```python
from build123d import *

# Parameters (mm, degrees)
EXTRUDE_1_DEPTH = 2697
SKETCH_2_W      = 61
SKETCH_2_H      = 134
EXTRUDE_2_DEPTH = 6
SKETCH_3_W      = 61
SKETCH_3_H      = 134
EXTRUDE_3_DEPTH = 6


with BuildPart() as part:
    # Model → 凸台-拉伸1 (new body)
    with BuildSketch(Plane.XY):
        with BuildLine():
            Line((11739.240027423, -58278.413223948), (11736.240027423, -58275.413223948))
            Line((11736.240027423, -58275.413223948), (11691.240027423, -58275.413223948))
            Line((11691.240027423, -58275.413223948), (11688.240027423, -58278.413223948))
            Line((11688.240027423, -58278.413223948), (11681.240027423, -58278.413223948))
            Line((11681.240027423, -58278.413223948), (11681.240027423, -58270.413223948))
            Line((11681.240027423, -58270.413223948), (11739.240027423, -58270.413223948))
            ThreePointArc((11739.240027423, -58270.413223948), (11741.361347766, -58269.534544291), (11742.240027423, -58267.413223948))
            Line((11742.240027423, -58267.413223948), (11742.240027423, -58139.413223948))
            ThreePointArc((11742.240027423, -58139.413223948), (11741.361347766, -58137.291903604), (11739.240027423, -58136.413223948))
            Line((11739.240027423, -58136.413223948), (11681.240027423, -58136.413223948))
            Line((11681.240027423, -58136.413223948), (11681.240027423, -58128.413223948))
            Line((11681.240027423, -58128.413223948), (11688.240027423, -58128.413223948))
            Line((11688.240027423, -58128.413223948), (11691.240027423, -58131.413223948))
            Line((11691.240027423, -58131.413223948), (11736.240027423, -58131.413223948))
            Line((11736.240027423, -58131.413223948), (11739.240027423, -58128.413223948))
            Line((11739.240027423, -58128.413223948), (11746.240027423, -58128.413223948))
            Line((11746.240027423, -58128.413223948), (11746.240027423, -58278.413223948))
            Line((11746.240027423, -58278.413223948), (11739.240027423, -58278.413223948))
        make_face()
    extrude(amount=EXTRUDE_1_DEPTH)

    # 草图2 → 凸台-拉伸2 (add)
    with BuildSketch(Plane.XY.offset(2697)):
        with Locations((11711.740027423, -58203.413223948)):
            Rectangle(SKETCH_2_W, SKETCH_2_H)
    extrude(amount=-EXTRUDE_2_DEPTH)

    # 草图3 → 凸台-拉伸3 (add)
    with BuildSketch(Plane(origin=(0, 0, 0), x_dir=(-1, 0, 0), z_dir=(0, 0, -1))):
        with Locations((-11711.740027423, -58203.413223948)):
            Rectangle(SKETCH_3_W, SKETCH_3_H)
    extrude(amount=-EXTRUDE_3_DEPTH)


solid = part.part
```
Design review of the part built by this model. Coordinates are the model's own, in mm. A direction names the side the tool comes from. Give positions to 0.01 mm unless a question says otherwise; leave off trailing zeros. Order: outer loops, then holes, each group sorted by start corner. A loop starts at its lowest first (then second) coordinate and runs counter-clockwise, first axis right, second up. Notation, with made-up numbers: (0, 83) -> (32, 83) arc R15 ccw to (32, 99) -> close; hole circle Ø1 at (71, 22). An arc over 180 degrees is marked (long way). Write item = value, one per line. Start each with the question number.
(1) We need section A-A on x = 11709. Write out the cut boundary in (y, z), plus the area to 3 significant figures.
(2) For faces 5 (the face through (11711, -58202, 2691)), 6 (the face through (11713, -58202, 2697)), 7 (the face through (11713, -58131.413, 1330)), list the 3-axis set-ups (+Z, -Z, +X, -X, +Y, -Y) from which the entire face can be reached by the end or side of a thin tool; tool diameter is ignored.
(3) For pin 1 (6 mm diameter, centred on x = 11724.5, z = 1025, fed in from +Y); pin 2 (1 mm diameter, centred on x = 11698.5, z = 894.5, fed in from -Y); pin 3 (8 mm diameter, centred on y = -58248, z = 2144.5, fed in from -X), all flat-tipped, find the tip position at first contact; note any pin that passes through.
(4) We need section C-C on z = 1862. Write out the cut boundary in (x, y), plus the area to 3 significant figures.
(5) We need section B-B on y = -58181. Write out the cut boundary in (x, z).
(6) Mouldability with a two-part tool opening along Y and no side actions: class faces 1 (the face through (11714, -58275.413, 1330)), 2 (the face through (11681.24, -58276, 1355)), 3 (the face through (11710, -58270.413, 1330)), 4 (the face through (11742.24, -58204, 1330)) as +Y half, -Y half, draft (parallel to the pull), parting line (faces both ways), or undercut.
(7) To check wall thickness, follow line 1 along Z through (x, y) = (11710, -58231.5); line 2 along Y through (x, z) = (11740.5, 1716.5); line 3 along Y through (x, z) = (11708, 1932). State the ranges of each line that lie inside material, in increasing order.
Numbers:
q1.outline = (-58275.41, 0) -> (-58131.41, 0) -> (-58131.41, 2697) -> (-58275.41, 2697) -> close; hole (-58270.41, 6) -> (-58136.41, 6) -> (-58136.41, 2691) -> (-58270.41, 2691) -> close
q1.area = 28,600 mm^2
q2.face_5 = -X
q2.face_6 = +Z, +X, -X, +Y, -Y
q2.face_7 = +Z, -Z, +Y
q3.pin_1 = -58131.41
q3.pin_2 = -58275.41
q3.pin_3 = 11742.24
q4.outline = (11681.24, -58278.41) -> (11688.24, -58278.41) -> (11691.24, -58275.41) -> (11736.24, -58275.41) -> (11739.24, -58278.41) -> (11746.24, -58278.41) -> (11746.24, -58128.41) -> (11739.24, -58128.41) -> (11736.24, -58131.41) -> (11691.24, -58131.41) -> (11688.24, -58128.41) -> (11681.24, -58128.41) -> (11681.24, -58136.41) -> (11739.24, -58136.41) arc R3 cw to (11742.24, -58139.41) -> (11742.24, -58267.41) arc R3 cw to (11739.24, -58270.41) -> (11681.24, -58270.41) -> close
q4.area = 1,290 mm^2
q5.outline = (11681.24, 0) -> (11746.24, 0) -> (11746.24, 2697) -> (11681.24, 2697) -> (11681.24, 2691) -> (11742.24, 2691) -> (11742.24, 6) -> (11681.24, 6) -> close
q6.face_1 = -Y half
q6.face_2 = draft
q6.face_3 = undercut
q6.face_4 = undercut
q7.line_1 = 0 to 6, 2691 to 2697
q7.line_2 = -58278.41 to -58270.14, -58136.69 to -58128.41
q7.line_3 = -58275.41 to -58270.41, -58136.41 to -58131.41
